Read the model definition and answer for the solid it produces. Units are mm, in the model's axes. Face numbers are marked on the shaded views. A direction names the side the tool comes from. Coordinates: 2 decimals unless noted, no trailing zeros. Write each loop counter-clockwise with the first axis right and the second up, starting at its lowest first coordinate (ties: lowest second). Pieces come first, ordered by that corner, then holes.
Item 1: Section B-B (z = 4.5) is taken. State how many separate pieces and enclosed holes the cut face has, then the cut area to 3 significant figures.
Item 2: Section A-A (x = 0) is taken. Give the vertices of the cut face in (y, z).
Item 3: Section D-D (x = 72) is taken. Give the vertices of the cut face in (y, z).
Item 4: Section C-C (x = 90) is taken. Give the vertices of the cut face in (y, z).
Item 5: Each of these flat-tipped pins is pushed along its axis until it touches: P1, Ø6, axis at y = -10, z = 9, coming from the +X side; P2, Ø6, axis at y = -34.5, z = 16, coming from the -X side; P3, Ø10, axis at x = -2.5, y = -19, coming from the -Z side; P4, Ø1, axis at x = 75.5, y = -20, coming from the -Z side. Where does it stop, or does it pass through?
Item 6: Determine the mould class of the marked faces 3, 4 and 5 for opening direction Z: released by +Z, released by -Z, zero draft, split by the parting line, or undercut.
Item 7: Straight lines are drawn through the part: probe 1 along Z at (x, y) = (0, -13); probe 2 along Y at (x, z) = (57.5, -1.5); probe 3 along Z at (x, y) = (90, -9). For each, find the intervals that lie inside material, in ascending order.
Item 8: A tool of negligible diameter and unlimited length cuts with its end or side. For the marked faces 1 and 2, from which of +Z, -Z, +X, -X, +Y, -Y can it reach the whole face along a straight path? Write none if from no direction.
from build123d import *

# Parameters (mm, degrees)
F0_R     = 10
F1_DEPTH = 25
F2_DEPTH = 50
F3_SIZE  = 2


with BuildPart() as f1:
    # F0 (on Front) → F1 (new body)
    with BuildSketch(Plane.XZ):
        with BuildLine():
            ThreePointArc((107.5, 0), (102.8684682655, 11.8597017037), (91.4254257714, 17.4418508585))
            ThreePointArc((91.4254257714, 17.4418508585), (72.5000007528, -0.0051329802), (91.4356573743, -17.4410116651))
            ThreePointArc((91.4356573743, -17.4410116651), (102.8719463185, -11.8559267025), (107.5, 0))
        make_face()
        with Locations((90, 0)):
            Circle(F0_R, mode=Mode.SUBTRACT)
        with BuildLine():
            ThreePointArc((4.9169029747, 24.5117128153), (19.3380786839, 15.8442012363), (25, 0))
            ThreePointArc((25, 0), (19.185007985, -16.0292067369), (4.4451625108, -24.6016367393))
            Line((4.4451625108, -24.6016367393), (91.4356573743, -17.4410116651))
            ThreePointArc((91.4356573743, -17.4410116651), (72.5000007528, -0.0051329802), (91.4254257714, 17.4418508585))
            Line((91.4254257714, 17.4418508585), (4.9169029747, 24.5117128153))
        make_face()
        with BuildLine():
            ThreePointArc((4.4451625108, -24.6016367393), (19.185007985, -16.0292067369), (25, 0))
            ThreePointArc((25, 0), (19.3380786839, 15.8442012363), (4.9169029747, 24.5117128153))
            ThreePointArc((4.9169029747, 24.5117128153), (-24.9988468465, 0.2401173553), (4.4451625108, -24.6016367393))
        make_face()
        Circle(F0_R, mode=Mode.SUBTRACT)
    extrude(amount=F1_DEPTH)

    # F0 (on Front) → F2 (join)
    with BuildSketch(Plane.XZ):
        with BuildLine():
            ThreePointArc((4.4451625108, -24.6016367393), (19.185007985, -16.0292067369), (25, 0))
            ThreePointArc((25, 0), (19.3380786839, 15.8442012363), (4.9169029747, 24.5117128153))
            ThreePointArc((4.9169029747, 24.5117128153), (-24.9988468465, 0.2401173553), (4.4451625108, -24.6016367393))
        make_face()
        Circle(F0_R, mode=Mode.SUBTRACT)
    extrude(amount=F2_DEPTH)

    # F3
    f3_edges = [f1.edges().sort_by_distance(p)[0] for p in [
        (-10, -50, 0),
        (-4.445163, -50, 24.601637),
        (80, -25, 0),
    ]]
    chamfer(f3_edges, length=F3_SIZE)


solid = f1.part
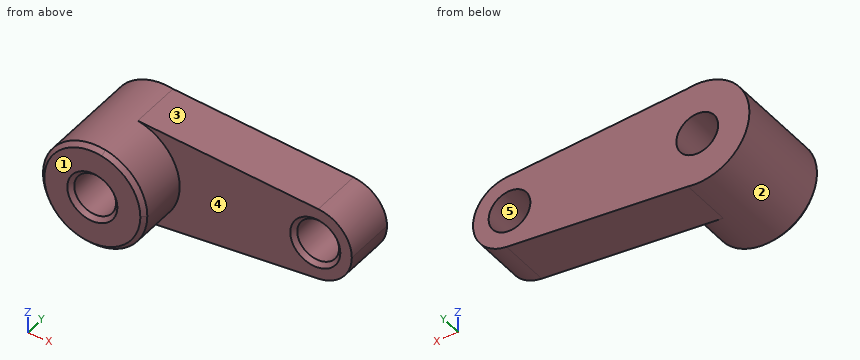
Established:
1. separate pieces: 3
1. enclosed holes: 0
1. area: 3,160 mm2
2. outline: (-50, -23) - (-48, -25) - (0, -25) - (0, -10) - (-48, -10) - (-50, -12) - close; (-50, 12) - (-48, 10) - (0, 10) - (0, 25) - (-48, 25) - (-50, 23) - close
3. outline: (-25, -19.04) - (0, -19.04) - (0, 19.03) - (-25, 19.03) - close
4. outline: (-25, -17.56) - (0, -17.56) - (0, -10) - (-23, -10) - (-25, -12) - close; (-25, 12) - (-23, 10) - (0, 10) - (0, 17.56) - (-25, 17.56) - close
5. P1: stops at x = 106.44
5. P2: stops at x = -21.35
5. P3: stops at z = -25
5. P4: stops at z = -18.79
6. face 3: released by +Z
6. face 4: zero draft
6. face 5: undercut
7. probe 1: z = -25 to -10, 10 to 25
7. probe 2: y = -25 to 0
7. probe 3: z = -17.56 to -10, 10 to 17.56
8. face 1: +Z, -Z, +X, -X, -Y
8. face 2: -Y
